from build123d import *

# Parameters (mm, degrees)
SKETCH_1_W          = 34
SKETCH_1_H          = 24
EXTRUDE_1_DEPTH     = 1
SKETCH_2_W          = 4
SKETCH_2_H          = 20
EXTRUDE_2_DEPTH     = 1
SKETCH_3_W          = 3.5
SKETCH_3_H          = 1.2
CUT_EXTRUDE_1_DEPTH = 25.207436874
FILLET_1_R          = 0.6
FILLET_2_R          = 0.5
FILLET_3_R          = 0.4
SKETCH_4_R          = 1.5
CUT_EXTRUDE_2_DEPTH = 25.207436874
SKETCH_8_W          = 20
SKETCH_8_H          = 20
EXTRUDE_9_DEPTH     = 2
SKETCH_5_W          = 22
SKETCH_5_H          = 22
EXTRUDE_3_DEPTH     = 3
SKETCH_6_W          = 1
SKETCH_6_H          = 22
CUT_EXTRUDE_3_DEPTH = 2
FILLET_4_R          = 0.5


# Some blends are built 0.0001 mm under size
with BuildPart() as part:
    # 草图1 → 凸台-拉伸1 (new body)
    with BuildSketch(Plane(origin=(0, 0, 0), x_dir=(1, 0, 0), z_dir=(0, 1, 0))):
        Rectangle(SKETCH_1_W, SKETCH_1_H)
    extrude(amount=EXTRUDE_1_DEPTH)

    # 草图2 → 凸台-拉伸2 (add)
    with BuildSketch(Plane(origin=(0, 0, 0), x_dir=(1, 0, 0), z_dir=(0, 1, 0))):
        with Locations((19, 0)):
            Rectangle(SKETCH_2_W, SKETCH_2_H)
    extrude(amount=EXTRUDE_2_DEPTH)

    # 草图3 → 切除-拉伸1 (cut, through all)
    with BuildSketch(Plane(origin=(0, 1, 0), x_dir=(1, 0, 0), z_dir=(0, 1, 0))):
        with Locations((19.25, -6.2)):
            Rectangle(SKETCH_3_W, SKETCH_3_H)
    extrude(amount=-CUT_EXTRUDE_1_DEPTH, mode=Mode.SUBTRACT)

    # 圆角1
    fillet_1_edges = [part.edges().sort_by_distance(p)[0] for p in [
        (17.5, 0.5, 6.8),
        (17.5, 0.5, 5.6),
    ]]
    fillet(fillet_1_edges, radius=FILLET_1_R - 0.0001)  # a hair under: the kernel refuses the full size

    # 圆角2
    fillet_2_edges = [part.edges().sort_by_distance(p)[0] for p in [
        (17, 0.5, -10),
        (17, 0.5, 10),
    ]]
    fillet(fillet_2_edges, radius=FILLET_2_R)

    # 圆角3
    fillet_3_edges = [part.edges().sort_by_distance(p)[0] for p in [
        (21, 0.5, 10),
        (21, 0.5, -10),
    ]]
    fillet(fillet_3_edges, radius=FILLET_3_R)

    # 草图4 → 切除-拉伸2 (cut, through all)
    with BuildSketch(Plane(origin=(0, 1, 0), x_dir=(1, 0, 0), z_dir=(0, 1, 0))):
        with Locations((-17, 7)):
            Circle(SKETCH_4_R)
    extrude(amount=-CUT_EXTRUDE_2_DEPTH, mode=Mode.SUBTRACT)

    # 草图8 → 凸台-拉伸9 (add)
    with BuildSketch(Plane(origin=(0, 1, 0), x_dir=(1, 0, 0), z_dir=(0, 1, 0))):
        with Locations((-2, -1)):
            Rectangle(SKETCH_8_W, SKETCH_8_H)
    extrude(amount=EXTRUDE_9_DEPTH)

    # 草图5 → 凸台-拉伸3 (add)
    with BuildSketch(Plane(origin=(0, 3, 0), x_dir=(1, 0, 0), z_dir=(0, 1, 0))):
        with Locations((-2, -1)):
            Rectangle(SKETCH_5_W, SKETCH_5_H)
    extrude(amount=EXTRUDE_3_DEPTH)

    # 草图6 → 切除-拉伸3 (cut)
    with BuildSketch(Plane(origin=(0, 6, 0), x_dir=(1, 0, 0), z_dir=(0, 1, 0))):
        with Locations((-2, -1)):
            Rectangle(SKETCH_6_W, SKETCH_6_H)
        with Locations((0, -1)):
            Rectangle(SKETCH_6_W, SKETCH_6_H)
        with Locations((2, -1)):
            Rectangle(SKETCH_6_W, SKETCH_6_H)
        with Locations((4, -1)):
            Rectangle(SKETCH_6_W, SKETCH_6_H)
        with Locations((6, -1)):
            Rectangle(SKETCH_6_W, SKETCH_6_H)
        with Locations((8, -1)):
            Rectangle(SKETCH_6_W, SKETCH_6_H)
        with Locations((-4, -1)):
            Rectangle(SKETCH_6_W, SKETCH_6_H)
        with Locations((-6, -1)):
            Rectangle(SKETCH_6_W, SKETCH_6_H)
        with Locations((-8, -1)):
            Rectangle(SKETCH_6_W, SKETCH_6_H)
        with Locations((-10, -1)):
            Rectangle(SKETCH_6_W, SKETCH_6_H)
        with Locations((-12, -1)):
            Rectangle(SKETCH_6_W, SKETCH_6_H)
    extrude(amount=-CUT_EXTRUDE_3_DEPTH, mode=Mode.SUBTRACT)

    # 圆角4
    # the kernel refuses this fillet: 0.5 mm, written as the material it takes off along each edge
    with BuildSketch(Plane(origin=(-13, 6, 13.25), x_dir=(0, -1, 0), z_dir=(0, 0, -1)), Plane(origin=(-11.5, 6, 13.25), x_dir=(0, -1, 0), z_dir=(0, 0, -1)), Plane(origin=(-9.5, 6, 13.25), x_dir=(0, -1, 0), z_dir=(0, 0, -1)), Plane(origin=(0.5, 6, 13.25), x_dir=(0, -1, 0), z_dir=(0, 0, -1)), Plane(origin=(2.5, 6, 13.25), x_dir=(0, -1, 0), z_dir=(0, 0, -1)), Plane(origin=(4.5, 6, 13.25), x_dir=(0, -1, 0), z_dir=(0, 0, -1)), Plane(origin=(6.5, 6, 13.25), x_dir=(0, -1, 0), z_dir=(0, 0, -1)), Plane(origin=(8.5, 6, 13.25), x_dir=(0, -1, 0), z_dir=(0, 0, -1)), Plane(origin=(-3.5, 6, 13.25), x_dir=(0, -1, 0), z_dir=(0, 0, -1)), Plane(origin=(-5.5, 6, 13.25), x_dir=(0, -1, 0), z_dir=(0, 0, -1)), Plane(origin=(-7.5, 6, 13.25), x_dir=(0, -1, 0), z_dir=(0, 0, -1)), Plane(origin=(-2.5, 6, 13.25), x_dir=(-1, 0, 0), z_dir=(0, 0, -1))) as fillet_4_piece_1:
        with BuildLine():
            CenterArc((FILLET_4_R, -FILLET_4_R), FILLET_4_R, 90, 90)
            Line((0, -FILLET_4_R), (0, 0))
            Line((0, 0), (FILLET_4_R, 0))
        make_face()
    extrude(amount=24.5, mode=Mode.SUBTRACT)
    with BuildSketch(Plane(origin=(-11.25, 6, 12), x_dir=(0, -1, 0), z_dir=(-1, 0, 0)), Plane(origin=(10.25, 6, 12), x_dir=(0, -1, 0), z_dir=(-1, 0, 0))) as fillet_4_piece_2:
        with BuildLine():
            CenterArc((FILLET_4_R, -FILLET_4_R), FILLET_4_R, 90, 90)
            Line((0, -FILLET_4_R), (0, 0))
            Line((0, 0), (FILLET_4_R, 0))
        make_face()
    extrude(amount=3, mode=Mode.SUBTRACT)
    with BuildSketch(Plane(origin=(9, 6, -11.25), x_dir=(-1, 0, 0), z_dir=(0, 0, 1)), Plane(origin=(-12.5, 6, -11.25), x_dir=(-1, 0, 0), z_dir=(0, 0, 1)), Plane(origin=(-10.5, 6, -11.25), x_dir=(-1, 0, 0), z_dir=(0, 0, 1)), Plane(origin=(-0.5, 6, -11.25), x_dir=(-1, 0, 0), z_dir=(0, 0, 1)), Plane(origin=(1.5, 6, -11.25), x_dir=(-1, 0, 0), z_dir=(0, 0, 1)), Plane(origin=(3.5, 6, -11.25), x_dir=(-1, 0, 0), z_dir=(0, 0, 1)), Plane(origin=(5.5, 6, -11.25), x_dir=(-1, 0, 0), z_dir=(0, 0, 1)), Plane(origin=(7.5, 6, -11.25), x_dir=(-1, 0, 0), z_dir=(0, 0, 1)), Plane(origin=(-4.5, 6, -11.25), x_dir=(-1, 0, 0), z_dir=(0, 0, 1)), Plane(origin=(-6.5, 6, -11.25), x_dir=(-1, 0, 0), z_dir=(0, 0, 1)), Plane(origin=(-8.5, 6, -11.25), x_dir=(-1, 0, 0), z_dir=(0, 0, 1)), Plane(origin=(-1.5, 6, -11.25), x_dir=(0, -1, 0), z_dir=(0, 0, 1))) as fillet_4_piece_3:
        with BuildLine():
            CenterArc((FILLET_4_R, FILLET_4_R), FILLET_4_R, 180, 90)
            Line((0, FILLET_4_R), (0, 0))
            Line((0, 0), (FILLET_4_R, 0))
        make_face()
    extrude(amount=24.5, mode=Mode.SUBTRACT)
    with BuildSketch(Plane(origin=(7.25, 6, -10), x_dir=(0, 0, 1), z_dir=(1, 0, 0)), Plane(origin=(-14.25, 6, -10), x_dir=(0, 0, 1), z_dir=(1, 0, 0))) as fillet_4_piece_4:
        with BuildLine():
            CenterArc((FILLET_4_R, FILLET_4_R), FILLET_4_R, 180, 90)
            Line((0, FILLET_4_R), (0, 0))
            Line((0, 0), (FILLET_4_R, 0))
        make_face()
    extrude(amount=3, mode=Mode.SUBTRACT)
    with BuildSketch(Plane(origin=(-9.25, 6, 12), x_dir=(0, -1, 0), z_dir=(-1, 0, 0)), Plane(origin=(-7.25, 6, 12), x_dir=(0, -1, 0), z_dir=(-1, 0, 0)), Plane(origin=(-5.25, 6, 12), x_dir=(0, -1, 0), z_dir=(-1, 0, 0)), Plane(origin=(-3.25, 6, 12), x_dir=(0, -1, 0), z_dir=(-1, 0, 0)), Plane(origin=(-1.25, 6, 12), x_dir=(0, -1, 0), z_dir=(-1, 0, 0)), Plane(origin=(0.75, 6, 12), x_dir=(0, -1, 0), z_dir=(-1, 0, 0)), Plane(origin=(2.75, 6, 12), x_dir=(0, -1, 0), z_dir=(-1, 0, 0)), Plane(origin=(4.75, 6, 12), x_dir=(0, -1, 0), z_dir=(-1, 0, 0)), Plane(origin=(6.75, 6, 12), x_dir=(0, -1, 0), z_dir=(-1, 0, 0)), Plane(origin=(8.75, 6, 12), x_dir=(0, -1, 0), z_dir=(-1, 0, 0))) as fillet_4_piece_5:
        with BuildLine():
            CenterArc((FILLET_4_R, -FILLET_4_R), FILLET_4_R, 90, 90)
            Line((0, -FILLET_4_R), (0, 0))
            Line((0, 0), (FILLET_4_R, 0))
        make_face()
    extrude(amount=3.5, mode=Mode.SUBTRACT)
    with BuildSketch(Plane(origin=(5.25, 6, -10), x_dir=(0, 0, 1), z_dir=(1, 0, 0)), Plane(origin=(3.25, 6, -10), x_dir=(0, 0, 1), z_dir=(1, 0, 0)), Plane(origin=(1.25, 6, -10), x_dir=(0, 0, 1), z_dir=(1, 0, 0)), Plane(origin=(-0.75, 6, -10), x_dir=(0, 0, 1), z_dir=(1, 0, 0)), Plane(origin=(-2.75, 6, -10), x_dir=(0, 0, 1), z_dir=(1, 0, 0)), Plane(origin=(-4.75, 6, -10), x_dir=(0, 0, 1), z_dir=(1, 0, 0)), Plane(origin=(-6.75, 6, -10), x_dir=(0, 0, 1), z_dir=(1, 0, 0)), Plane(origin=(-8.75, 6, -10), x_dir=(0, 0, 1), z_dir=(1, 0, 0)), Plane(origin=(-10.75, 6, -10), x_dir=(0, 0, 1), z_dir=(1, 0, 0)), Plane(origin=(-12.75, 6, -10), x_dir=(0, 0, 1), z_dir=(1, 0, 0))) as fillet_4_piece_6:
        with BuildLine():
            CenterArc((FILLET_4_R, FILLET_4_R), FILLET_4_R, 180, 90)
            Line((0, FILLET_4_R), (0, 0))
            Line((0, 0), (FILLET_4_R, 0))
        make_face()
    extrude(amount=3.5, mode=Mode.SUBTRACT)


solid = part.part
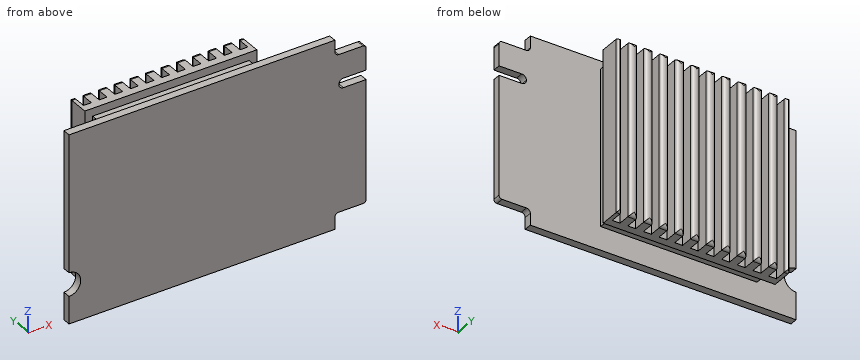
Read the model definition and answer for the solid it produces. Units are mm, in the model's axes. Coordinates: 2 decimals unless noted, no trailing zeros. Order: outer loops, then holes, each group sorted by start corner. A loop starts at its lowest first (then second) coordinate and runs counter-clockwise, first axis right, second up. Notation, with made-up numbers: (49, 62.5) - (86, 62.5) arc R31 ccw to (86, 93.5) - close; hole circle Ø3 at (-18.75, -12.5). An arc over 180 degrees is marked (long way). Use one line per item in the form item = value.
(1) Section C-C, the plane y = 2.6 is taken. Give the vertices of the cut face in (x, z), then the cut area to 3 significant figures.
Computed values:
outline = (-12, -9) - (8, -9) - (8, 11) - (-12, 11) - close
area = 400 mm²
(2) Straight lines are drawn through the part: L1, parallel to Y at x = -12, z = -9.75; L2, parallel to Y at x = -11, z = 11.25; L3, parallel to Z at x = 1, y = 3.8. For each, find the intervals that lie inside material, in ascending order.
Computed values:
L1 = 0 to 1, 3 to 4
L2 = 0 to 1, 3 to 6
L3 = -10 to 12
(3) Section D-D, the plane x = 10 is taken. Give the vertices of the cut face in (y, z).
Computed values:
outline = (0, -12) - (1, -12) - (1, 12) - (0, 12) - close
(4) Section A-A, the plane x = -6 is taken. Give the vertices of the cut face in (y, z), then the cut area to 3 significant figures.
Computed values:
outline = (0, -12) - (1, -12) - (1, -9) - (3, -9) - (3, -10) - (4, -10) - (4, 12) - (3, 12) - (3, 11) - (1, 11) - (1, 12) - (0, 12) - close
area = 86.0 mm²
(5) Section B-B, the plane y = 4.6 is taken. Give the number of separate pieces and of enclosed holes in the cut face, then the cut area to 3 significant figures.
Computed values:
separate_pieces = 12
enclosed_holes = 0
area = 242 mm²
(6) Given pin 1 Ø0.8 at (y, z) = (0.5, 11) entering from +X; pin 2 Ø0.8 at (y, z) = (4.5, 6) entering from +X; pin 3 Ø2 at (x, z) = (13.5, -4.5) entering from +Y, each flat-ended and moving along its own axis, determine where each tip first touches the part or whether it passes through.
Computed values:
pin_1 = 17
pin_2 = 9
pin_3 = 1
